from build123d import *

# Parameters (mm, degrees)
F1_DEPTH = 0.35
F2_DEPTH = 0.5


with BuildPart() as f1:
    # F0 (on Front) → F1 (new body)
    with BuildSketch(Plane.XZ):
        with BuildLine():
            Line((-190.517892, -51.960177), (-190.517892, -29.210177))
            Line((-190.517892, -29.210177), (-252.517892, -29.210177))
            Line((-252.517892, -29.210177), (-252.517892, -51.960177))
            Line((-252.517892, -51.960177), (-240.517892, -51.960177))
            ThreePointArc((-240.517892, -51.960177), (-221.517892, -32.960177), (-202.517892, -51.960177))
            Line((-202.517892, -51.960177), (-190.517892, -51.960177))
        make_face()
    extrude(amount=F1_DEPTH)

    # F0 (on Front) → F2 (join)
    with BuildSketch(Plane.XZ):
        with BuildLine():
            Line((-206.017892, -51.960177), (-202.517892, -51.960177))
            ThreePointArc((-202.517892, -51.960177), (-221.517892, -32.960177), (-240.517892, -51.960177))
            Line((-240.517892, -51.960177), (-237.017892, -51.960177))
            ThreePointArc((-237.017892, -51.960177), (-221.517892, -36.460177), (-206.017892, -51.960177))
        make_face()
    extrude(amount=F2_DEPTH)


solid = f1.part
Verification items for the finished model (mm, model axes). A direction names the side the tool comes from. Give positions to 0.01 mm unless a question says otherwise; leave off trailing zeros. Loops run counter-clockwise (first coordinate to the right, second up) from the corner with the lowest first, then second, coordinate; pieces in that order, holes last.
1. Material ranges on probe 1 along Y at (x, z) = (-234.5, -35); probe 2 along X at (y, z) = (-0.3, -49.25); probe 3 along X at (y, z) = (-0.2, -49.5), recorded low to high.
Derived:
probe 1: y = -0.35 to 0
probe 2: x = -252.52 to -236.78, -206.26 to -190.52
probe 3: x = -252.52 to -236.82, -206.21 to -190.52
2. Cross-section at C-C on x = -244. Record the cut outline in (y, z), and give its area (3 significant figures).
Derived:
outline: (-0.35, -51.96) - (0, -51.96) - (0, -29.21) - (-0.35, -29.21) - close
area: 7.96 mm2
3. Cross-section at D-D on z = -31.75. Record the cut outline in (x, y).
Derived:
outline: (-252.52, -0.35) - (-190.52, -0.35) - (-190.52, 0) - (-252.52, 0) - close
4. Release check for a two-part mould opening along X. For faces 1 (the flat face through (-223, -0.5, -36)), 2 (the cylindrical face through (-221.859, -0.246, -36.464)) record: +X half, -X half, draft (parallel to the pull), parting line (faces both ways), or undercut.
Derived:
face 1: draft
face 2: undercut
5. Cross-section at B-B on y = -0.25. Record the cut outline in (x, z).
Derived:
outline: (-252.52, -51.96) - (-237.02, -51.96) arc R15.5 cw to (-206.02, -51.96) - (-190.52, -51.96) - (-190.52, -29.21) - (-252.52, -29.21) - close
6. Tool access check on faces 3 (the flat face through (-222, 0, -35)), 4 (the flat face through (-222, -0.35, -32.8)). Record the directions out of +Z, -Z, +X, -X, +Y, -Y that give a thin tool (end or side, any length) a straight path to the whole face; none if there is none.
Derived:
face 3: +Z, -Z, +X, -X, +Y
face 4: +Z, -Y
7. Cross-section at A-A on z = -40. Record the cut outline in (x, y), and give its area (3 significant figures).
Derived:
outline: (-252.52, -0.35) - (-236.28, -0.35) - (-236.28, -0.5) - (-231.38, -0.5) - (-231.38, 0) - (-252.52, 0) - close; (-211.66, -0.5) - (-206.75, -0.5) - (-206.75, -0.35) - (-190.52, -0.35) - (-190.52, 0) - (-211.66, 0) - close
area: 16.3 mm2
